Check sheet for the modelled part. Datum: model origin and axes. Units: mm. Round coordinates to 2 decimals unless told otherwise and drop trailing zeros. Write each loop counter-clockwise with the first axis right and the second up, starting at its lowest first coordinate (ties: lowest second). Pieces come first, ordered by that corner, then holes. Notation, with made-up numbers: (44, -31.75) -> (103, -31.75) arc R21 ccw to (103, -2.75) -> close; hole circle Ø11 at (-11.5, 8.25). An arc over 180 degrees is marked (long way). One line per item, written item: value.
from build123d import *

# Parameters (mm, degrees)
SKETCH2_W           = 250
SKETCH2_H           = 250
BOSS_EXTRUDE1_DEPTH = 3.175
SKETCH3_W           = 8.6
SKETCH3_H           = 15.35
CUT_EXTRUDE1_DEPTH  = 10
SKETCH4_W           = 45.1
SKETCH4_H           = 25.1
SKETCH4_W_2         = 25.1
SKETCH4_H_2         = 45.1
CUT_EXTRUDE2_DEPTH  = 10
M3_TAPPED_HOLE1_D   = 2.5
M3_TAPPED_HOLE2_D   = 2.5


with BuildPart() as part:
    # Sketch2 → Boss-Extrude1 (new body)
    with BuildSketch(Plane(origin=(0, 0, 0), x_dir=(1, 0, 0), z_dir=(0, 1, 0))):
        Rectangle(SKETCH2_W, SKETCH2_H)
    extrude(amount=BOSS_EXTRUDE1_DEPTH)

    # Sketch3 → Cut-Extrude1 (cut)
    with BuildSketch(Plane(origin=(0, 3.175, 0), x_dir=(1, 0, 0), z_dir=(0, 1, 0))):
        with Locations((-43.75, 35.675)):
            Rectangle(SKETCH3_W, SKETCH3_H)
        with Locations((-43.75, -35.675)):
            Rectangle(SKETCH3_W, SKETCH3_H)
        with Locations((43.75, -35.675)):
            Rectangle(SKETCH3_W, SKETCH3_H)
        with Locations((43.75, 35.675)):
            Rectangle(SKETCH3_W, SKETCH3_H)
    extrude(amount=-CUT_EXTRUDE1_DEPTH, mode=Mode.SUBTRACT)

    # Sketch4 → Cut-Extrude2 (cut)
    with BuildSketch(Plane(origin=(0, 3.175, 0), x_dir=(1, 0, 0), z_dir=(0, 1, 0))):
        with Locations((0, 125)):
            Rectangle(SKETCH4_W, SKETCH4_H)
        with Locations((125, 0)):
            Rectangle(SKETCH4_W_2, SKETCH4_H_2)
        with Locations((0, -125)):
            Rectangle(SKETCH4_W, SKETCH4_H)
        with Locations((-125, 0)):
            Rectangle(SKETCH4_W_2, SKETCH4_H_2)
    extrude(amount=-CUT_EXTRUDE2_DEPTH, mode=Mode.SUBTRACT)

    # M3 Tapped Hole1 (through all)
    with Locations(Plane(origin=(0, 3.175, 0), x_dir=(1, 0, 0), z_dir=(0, 1, 0))):
        with Locations((-115, 115)):
            Hole(M3_TAPPED_HOLE1_D / 2)

    # M3 Tapped Hole2 (through all)
    with Locations(Plane(origin=(0, 3.175, 0), x_dir=(1, 0, 0), z_dir=(0, 1, 0))):
        with Locations((115, 115), (115, -115), (-115, -115)):
            Hole(M3_TAPPED_HOLE2_D / 2)


solid = part.part
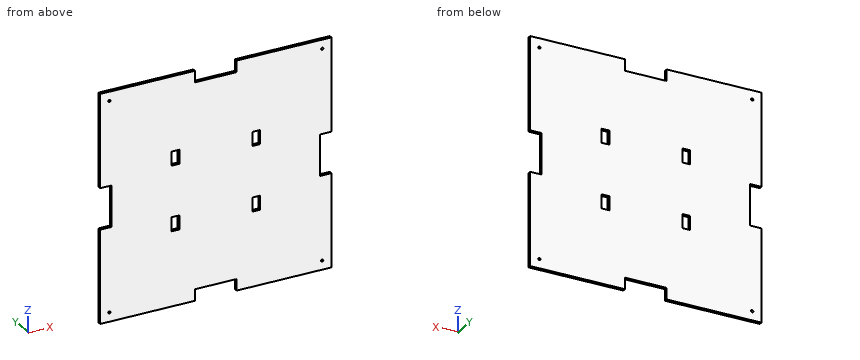
Item 1: Sectioned sample at A-A on x = -12. Enter the section's corners in (y, z) (3 decimals).
Answer:
outline: (0, -112.45) -> (3.175, -112.45) -> (3.175, 112.45) -> (0, 112.45) -> close
Item 2: Sectioned sample at B-B on y = 1.95. Count the separate pieces of the cut face and the enclosed holes in it, and give its area (3 significant figures).
Answer:
separate pieces: 1
enclosed holes: 8
area: 59,700 mm^2
Item 3: Thickness scan on line 1 (Z direction, x = -115, y = 1); line 2 (X direction, y = 1.4, z = -40). Record the ranges inside material, lowest first.
Answer:
line 1: z = -125 to -116.25, -113.75 to -22.55, 22.55 to 113.75, 116.25 to 125
line 2: x = -125 to -48.05, -39.45 to 39.45, 48.05 to 125
Item 4: Depth check by flat-ended pin: P1, Ø2, axis at x = 115, z = -115, coming from the -Y side; P2, Ø1, axis at x = 1.5, y = 1.5, coming from the +Z side. Enter the tip coordinate at first touch or a pass-through.
Answer:
P1: passes through
P2: stops at z = 112.45
